Answer from the drawing. Dimensions are ordinates in mm from the lowest x, y and z of the part. A direction names the side the tool comes from. Coordinates: 2 decimals unless noted, no trailing zeros. Write each loop counter-clockwise with the first axis right and the second up, starting at its lowest first coordinate (ties: lowest second). Pieces come first, ordered by that corner, then holes. Notation, with made-up numbers: (-29.75, 25.25) -> (11.25, 25.25) arc R17 cw to (11.25, 39.25) -> close; hole circle Ø1 at (34, -2.5). An arc over 180 degrees is marked (long way). Return JSON: item names as keys, results as strings.
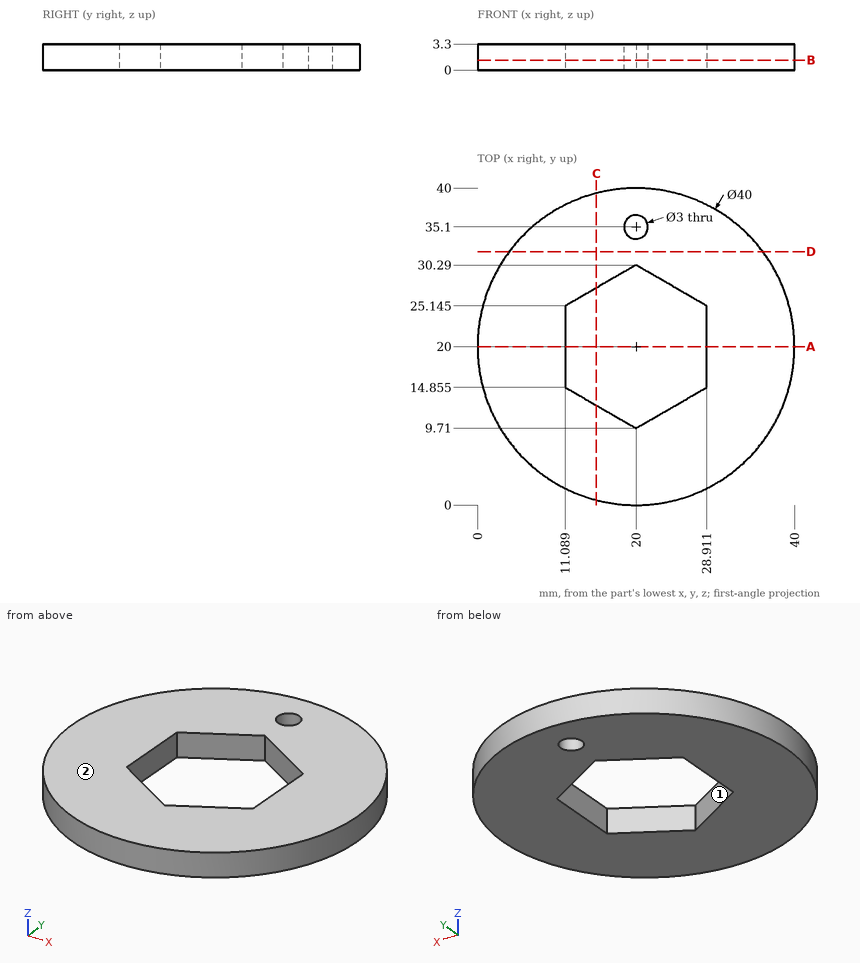
1. The part is cut by section B-B (z = 1.25). Determine the outline of the cut face in (x, y) (1 decimal).
Taken from the geometry:
{"outline": "circle Ø40 at (20, 20); hole (11.1, 14.9) -> (20, 9.7) -> (28.9, 14.9) -> (28.9, 25.1) -> (20, 30.3) -> (11.1, 25.1) -> close; hole circle Ø3 at (20, 35.1)"}
2. The part is cut by section C-C (x = 15). Determine the outline of the cut face in (y, z) (1 decimal).
Taken from the geometry:
{"outline": "(0.6, 0) -> (12.6, 0) -> (12.6, 3.3) -> (0.6, 3.3) -> close; (27.4, 0) -> (39.4, 0) -> (39.4, 3.3) -> (27.4, 3.3) -> close"}
3. A tool of negligible diameter and unlimited length cuts with its end or side. For the marked faces 1 and 2, from which of +Z, -Z, +X, -X, +Y, -Y can it reach the whole face along a straight path? Write none if from no direction.
Taken from the geometry:
{"face 1": "+Z, -Z", "face 2": "+Z, +X, -X, +Y, -Y"}
4. Flat-ended cylindrical pins translate along their axes: pin 1 Ø1 at (y, z) = (19, 1) entering from +X; pin 2 Ø1 at (y, z) = (19, 1) entering from -X; pin 3 Ø1 at (x, z) = (8, 1.5) entering from -Y. Find the tip coordinate at first contact, or state that the pin passes through.
Taken from the geometry:
{"pin 1": "stops at x = 39.99", "pin 2": "stops at x = 0.01", "pin 3": "stops at y = 3.64"}
5. The part is cut by section A-A (y = 20). Determine the outline of the cut face in (x, z).
Taken from the geometry:
{"outline": "(0, 0) -> (11.09, 0) -> (11.09, 3.3) -> (0, 3.3) -> close; (28.91, 0) -> (40, 0) -> (40, 3.3) -> (28.91, 3.3) -> close"}
6. Consider L1, parallel to Y at x = 20, z = 2.2; L2, parallel to X at y = 34, z = 3.1 (1 decimal); L3, parallel to X at y = 13.5, z = 2.9 (1 decimal). Determine where each line is inside the solid, lowest interval first.
Taken from the geometry:
{"L1": "y = 0 to 9.71, 30.29 to 33.6, 36.6 to 40", "L2": "x = 5.7 to 19, 21 to 34.3", "L3": "x = 1.1 to 13.4, 26.6 to 38.9"}
7. The part is cut by section D-D (y = 32). Determine the outline of the cut face in (x, z).
Taken from the geometry:
{"outline": "(4, 0) -> (36, 0) -> (36, 3.3) -> (4, 3.3) -> close"}
